For this review, take the finished solid that the model builds, in its own axes (mm). A direction names the side the tool comes from. Coordinates: 2 decimals unless noted, no trailing zeros. Loops run counter-clockwise (first coordinate to the right, second up) from the corner with the lowest first, then second, coordinate; pieces in that order, holes last. Notation, with made-up numbers: (-40, -3.75) -> (-9, -3.75) arc R27 cw to (-9, 13.25) -> close; hole circle Ø1 at (45.25, 38). An arc over 180 degrees is marked (long way). Answer in a Markdown table with one row per item.
from build123d import *

# Parameters (mm, degrees)
F1_DEPTH      = 3
F2_DEPTH      = 2
F4_DEPTH      = 2
F5_DEPTH      = 4
F7_DEPTH      = 2
F9_ANGLE      = 180
F10_T         = 2
F10_T4_ANGLE  = 180.000000001
F10_T6_ANGLE  = 180.000000001
F10_T8_ANGLE  = 180.000000001
F10_T10_ANGLE = 180.000000001
F11_DEPTH     = 3
F12_DEPTH     = 1
F13_DEPTH     = 3


# Not quite as in the source:
# - a shell that OpenCascade refuses in one call is made with other operations: the cavity is built on its own and cut out


with BuildPart() as f1:
    # F0 (on Front) → F1 (new body)
    with BuildSketch(Plane.XZ):
        with BuildLine():
            Line((15, 0), (-15, 0))
            ThreePointArc((-15, 0), (0, -15), (15, 0))
        make_face()
    extrude(amount=-F1_DEPTH)

    # F0 (on Front) → F2 (join)
    with BuildSketch(Plane.XZ):
        with BuildLine():
            ThreePointArc((15, 0), (0, -15), (-15, 0))
            Line((-15, 0), (-30, 0))
            ThreePointArc((-30, 0), (0, -30), (30, 0))
            Line((30, 0), (15, 0))
        make_face()
        with BuildLine():
            Line((15, 0), (-15, 0))
            ThreePointArc((-15, 0), (0, -15), (15, 0))
        make_face()
    extrude(amount=F2_DEPTH)

    # F3 (on face) → F4 (join)
    with BuildSketch(Plane.XZ.offset(2)):
        with BuildLine():
            ThreePointArc((-27, 0), (0, -27), (27, 0))
            Line((27, 0), (24, 0))
            ThreePointArc((24, 0), (0, -24), (-24, 0))
            Line((-24, 0), (-27, 0))
        make_face()
    extrude(amount=F4_DEPTH)

    # F5 (add): a face of the model
    f5_faces = [f1.faces().sort_by_distance(p)[0] for p in [
        (0, -2, -10.1859163579),
    ]]
    extrude(f5_faces, amount=F5_DEPTH)

    # F6 (on face) → F7 (join)
    with BuildSketch(Plane.XZ.offset(6)):
        with BuildLine():
            ThreePointArc((-21, 0), (0, -21), (21, 0))
            Line((21, 0), (-21, 0))
        make_face()
    extrude(amount=F7_DEPTH)

    # F8 (on face) → F9 (revolve)
    with BuildSketch(Plane.XY):
        with BuildLine():
            Line((0, -8), (-21, -8))
            ThreePointArc((-21, -8), (-11.8972036761, -16.2165961892), (0, -19.1881107091))
            Line((0, -19.1881107091), (0, -8))
        make_face()
    revolve(axis=Axis((0, 0.2930196971, 0), (0, -1, 0)), revolution_arc=F9_ANGLE)

    # F10: shell of thickness 2, made by hand


with BuildPart() as f10_core1:
    # F10_t2: copy of F1
    add(f1.part)

    # the walls: a layer under each face that stays
    f10_faces = [f10_core1.faces().sort_by_distance(p)[0] for p in [
        (0, -1, -30),
        (-20, 0, -15),
        (-25.7142857143, -2, -15),
        (0, -3, -27),
        (-23.1428571429, -4, -13.5),
        (0, -5, -24),
        (-20.5714285714, -6, -12),
        (0, -7, -21),
        (0, 1.5, -15),
        (0, 3, -7.5),
        (0, -16.2165961892, -11.8972036761),
    ]]
    thicken(f10_faces, amount=-F10_T, mode=Mode.SUBTRACT)

    # F10_s3 → F10_t4 (revolve, cut)
    with BuildSketch(Plane.XY):
        Polygon((-15.02, 0.02), (-15, -2), (-13, -2), (-13, 0), align=None)
    revolve(axis=Axis((0, 0, 0), (0, -1, 0)), revolution_arc=F10_T4_ANGLE, mode=Mode.SUBTRACT)

    # F10_s5 → F10_t6 (revolve, cut)
    with BuildSketch(Plane.XY):
        Polygon((-27.02, -2.02), (-27, 0), (-25, 0), (-25, -2), align=None)
    revolve(axis=Axis((0, -2, 0), (0, -1, 0)), revolution_arc=F10_T6_ANGLE, mode=Mode.SUBTRACT)

    # F10_s7 → F10_t8 (revolve, cut)
    with BuildSketch(Plane.XY):
        Polygon((24.02, -4.02), (24, -2), (22, -2), (22, -4), align=None)
    revolve(axis=Axis((0, -4, 0), (0, 1, 0)), revolution_arc=F10_T8_ANGLE, mode=Mode.SUBTRACT)

    # F10_s9 → F10_t10 (revolve, cut)
    with BuildSketch(Plane.XY):
        Polygon((-21.02, -6.02), (-21, -4), (-19, -4), (-19, -6), align=None)
    revolve(axis=Axis((0, -6, 0), (0, -1, 0)), revolution_arc=F10_T10_ANGLE, mode=Mode.SUBTRACT)


with BuildPart() as f1_1:
    add(f1.part)

    # what is left inside the walls is the cavity
    f10_cavity = [f10_core1.part.solids().sort_by_distance(p)[0] for p in [
        (0, -12.621798, -13.821356),
    ]]
    add(f10_cavity, mode=Mode.SUBTRACT)

    # F11 (add, through all): a face of the model
    f11_faces = [f1_1.faces().sort_by_distance(p)[0] for p in [
        (0, 1, -5.5173713605),
    ]]
    extrude(f11_faces, amount=F11_DEPTH)

    # F12 (cut): a face of the model
    f12_faces = [f1_1.faces().sort_by_distance(p)[0] for p in [
        (0, -2, -9.3370899946),
    ]]
    extrude(f12_faces, amount=-F12_DEPTH, mode=Mode.SUBTRACT)

    # F13 (add): a face of the model
    f13_faces = [f1_1.faces().sort_by_distance(p)[0] for p in [
        (0, -1, -9.3370899946),
    ]]
    extrude(f13_faces, amount=F13_DEPTH)


solid = f1_1.part
Item 1: Take a section at D-D, the plane z = -6. State the section outline as (x, y) points.
Worked answers:
| item | result |
|---|---|
| outline | (-29.39, -2) -> (-26.32, -2) -> (-26.32, -4) -> (-23.24, -4) -> (-23.24, -6) -> (-20.12, -6) -> (-20.12, -8) arc R24.58 ccw to (20.12, -8) -> (20.12, -6) -> (23.24, -6) -> (23.24, -4) -> (26.32, -4) -> (26.32, -2) -> (29.39, -2) -> (29.39, 0) -> (13.75, 0) -> (13.75, 3) -> (-13.75, 3) -> (-13.75, 0) -> (-29.39, 0) -> close; hole (-18.03, -7.38) arc R22.52 ccw to (18.03, -7.38) -> (18.03, -4) -> (-18.03, -4) -> close |
Item 2: The part is to be moulded in two halves that separate along Y. For faces 1 (the flat face through (0, 3, -6)), 2 (the cylindrical face through (0, 1, -15)), 3 (the flat face through (0, -4, -7)), 4 (the cylindrical face through (0, -6, -19)), say which applies: +Y half, -Y half, draft (parallel to the pull), parting line (faces both ways), or undercut.
Worked answers:
| item | result |
|---|---|
| face 1 | +Y half |
| face 2 | draft |
| face 3 | undercut |
| face 4 | undercut |
Item 3: Take a section at A-A, the plane z = -11. State the section outline as (x, y) points.
Worked answers:
| item | result |
|---|---|
| outline | (-27.91, -2) -> (-24.66, -2) -> (-24.66, -4) -> (-21.33, -4) -> (-21.33, -6) -> (-17.89, -6) -> (-17.89, -8) arc R22.79 ccw to (17.89, -8) -> (17.89, -6) -> (21.33, -6) -> (21.33, -4) -> (24.66, -4) -> (24.66, -2) -> (27.91, -2) -> (27.91, 0) -> (10.2, 0) -> (10.2, 3) -> (-10.2, 3) -> (-10.2, 0) -> (-27.91, 0) -> close; hole (-15.49, -7.38) arc R20.54 ccw to (15.49, -7.38) -> (15.49, -4) -> (-15.49, -4) -> close |
Item 4: Insertion check: pin 1 (5.5 mm diameter, centred on x = 7.5, z = -7, fed in from -Y); pin 2 (4 mm diameter, centred on y = -0.5, z = -12, fed in from +X); pin 3 (6 mm diameter, centred on y = -1.5, z = -12, fed in from +X). Each pin has a flat end and moves straight along its axis. Give the tip position at first contact, or say it passes through.
Worked answers:
| item | result |
|---|---|
| pin 1 | y = -18.05 |
| pin 2 | x = 28.28 |
| pin 3 | x = 28.62 |
Item 5: Take a section at C-C, the plane y = 0.75. State the section outline as (x, z) points, and give its area (3 significant figures).
Worked answers:
| item | result |
|---|---|
| outline | (-15, 0) arc R15 ccw to (15, 0) -> close |
| area | 353 mm² |
Item 6: For L1, parallel to Z at x = -0.5, y = -0.25; L2, parallel to Y at x = -1.5, z = -5.5; L3, parallel to X at y = -9.75, z = -5.5, list the stretches that pass through material, from the lowest coordinate up.
Worked answers:
| item | result |
|---|---|
| L1 | -30 to 0 |
| L2 | -18.54 to -16.48, -4 to 3 |
| L3 | -18.93 to -16.16, 16.16 to 18.93 |
Item 7: For faces 5 (the cylindrical face through (-0.594, -2.986, -26.993)), 6 (the cylindrical face through (-0.66, -0.986, -29.993)), 7 (the flat face through (0, 0, -18)), list the 3-axis set-ups (+Z, -Z, +X, -X, +Y, -Y) from which the entire face can be reached by the end or side of a thin tool; tool diameter is ignored.
Worked answers:
| item | result |
|---|---|
| face 5 | -Z, -Y |
| face 6 | -Z, +Y, -Y |
| face 7 | -Z, +Y |
Item 8: Take a section at B-B, the plane x = 0. State the section outline as (y, z) points.
Worked answers:
| item | result |
|---|---|
| outline | (-19.19, 0) arc R25.3 ccw to (-8, -21) -> (-6, -21) -> (-6, -24) -> (-4, -24) -> (-4, -27) -> (-2, -27) -> (-2, -30) -> (0, -30) -> (0, -15) -> (3, -15) -> (3, 0) -> (-4, 0) -> (-4, -19) -> (-7.38, -19) arc R23.3 cw to (-17.19, 0) -> close |
